Model file for the job. Use its own axes, mm. A direction names the side the tool comes from. Coordinates: 2 decimals unless noted, no trailing zeros. Write each loop counter-clockwise with the first axis right and the second up, starting at its lowest first coordinate (ties: lowest second). Pieces come first, ordered by that corner, then holes. Notation, with made-up numbers: M 51.5,56.5 L 104.5,56.5 A21 ccw 104.5,76.5 Z; hole C 51.5,-25 d11. An arc over 180 degrees is marked long. One line per question, with ' | ' between items. Start each with the question number.
(1) Flat gauge pins, fed straight in: pin 1 Ø6 at (y, z) = (-5, 5) entering from +X; pin 2 Ø1.5 at (y, z) = (-6.5, 5) entering from +X. Where does each tip first touch, or does it go through?
(2) Cut at A-A (x = 8). Write the cut outline in (y, z).
(3) Cut at D-D (z = 1.5). Write the cut outline in (x, y), plus the area to 3 significant figures.
(4) Two-plate mould, pull along Z, no slides. Class faces 3 (the face through (-6, -10, 5)), 4 (the face through (0, -5, 10)), 5 (the face through (-6.04, -3.66, 7.11)): +Z half, -Z half, draft (parallel to the pull), parting line (faces both ways), or undercut.
(5) Wall check: probe 1 along Y at (x, z) = (5, 5); probe 2 along Z at (x, y) = (0, -6.6); probe 3 along X at (y, z) = (-8.5, 6.25). Give the ranges that are in metal, low to high.
(6) Tool access for faces 1 (the face through (1.34, -2.85, 7.11)), 2 (the face through (-10, -3, 3)): list every direction of +Z, -Z, +X, -X, +Y, -Y with a clear straight run to the whole face (end or side of a thin tool).
(7) Cut at B-B (z = 5). Write the cut outline in (x, y), plus the area to 3 significant figures.
(8) Cut at C-C (y = -3.25). Write the cut outline in (x, z), plus the area to 3 significant figures.
from build123d import *

# Parameters (mm, degrees)
F0_W          = 20
F0_H          = 10
F1_DEPTH      = 10
F2_R          = 2.5
F3_DEPTH      = 8
F4_R          = 2.5
F5_DEPTH      = 10.001
F5_DEPTH_BACK = 10.001
F6_T1_DEPTH   = 35


# Not quite as in the source:
# - a fillet or chamfer that OpenCascade refuses, or shapes differently, is made with other operations: its cross-section is extruded or revolved along the edge and cut away or added


with BuildPart() as f1:
    # F0 (on Front) → F1 (new body)
    with BuildSketch(Plane.XZ):
        with Locations((0, 5)):
            Rectangle(F0_W, F0_H)
    extrude(amount=F1_DEPTH)

    # F2 (on face) → F3 (cut)
    with BuildSketch(Plane.XZ.offset(10)):
        with Locations((0, 5)):
            Circle(F2_R)
    extrude(amount=-F3_DEPTH, mode=Mode.SUBTRACT)

    # F4 (on Right) → F5 (cut, two sides)
    with BuildSketch(Plane.YZ) as f5_sk:
        with Locations((-5, 5)):
            Circle(F4_R)
    extrude(amount=-F5_DEPTH, mode=Mode.SUBTRACT)
    extrude(f5_sk.sketch, amount=F5_DEPTH_BACK, mode=Mode.SUBTRACT)

    # F6: fillet of radius 3 on 4 edges, made by hand

    # F6_s2 → F6_t1 (cut)
    with BuildSketch(Plane.YZ.offset(-17.5)):
        with BuildLine():
            ThreePointArc((-3, 10), (-0.8786796564, 9.1213203436), (0, 7))
            Line((0, 7), (0, 10))
            Line((0, 10), (-3, 10))
        make_face()
        with BuildLine():
            ThreePointArc((-7, 10), (-9.1213203436, 9.1213203436), (-10, 7))
            Line((-10, 7), (-10, 10))
            Line((-10, 10), (-7, 10))
        make_face()
        with BuildLine():
            ThreePointArc((-10, 3), (-9.1213203436, 0.8786796564), (-7, 0))
            Line((-7, 0), (-10, 0))
            Line((-10, 0), (-10, 3))
        make_face()
        with BuildLine():
            ThreePointArc((0, 3), (-0.8786796564, 0.8786796564), (-3, 0))
            Line((-3, 0), (0, 0))
            Line((0, 0), (0, 3))
        make_face()
    extrude(amount=F6_T1_DEPTH, mode=Mode.SUBTRACT)


solid = f1.part
Filled in:
1) pin 1: x = 10 | pin 2: through
2) outline: M -10,3 A3 ccw -7,0 L -3,0 A3 ccw 0,3 L 0,7 A3 ccw -3,10 L -7,10 A3 ccw -10,7 Z; hole C -5,5 d5
3) outline: M -10,-9.6 L 10,-9.6 L 10,-0.4 L -10,-0.4 Z | area: 184 mm²
4) face 3: draft | face 4: +Z half | face 5: undercut
5) probe 1: -10 to -7.5, -2.5 to 0 | probe 2: 0 to 2.5, 7.5 to 10 | probe 3: -10 to -2.17, 2.17 to 10
6) face 1: -Y | face 2: +Z, -Z, -X, +Y, -Y
7) outline: M -10,-10 L -2.5,-10 L -2.5,-7.5 L -10,-7.5 Z; M -10,-2.5 L -2.5,-2.5 L -2.5,-2 L 2.5,-2 L 2.5,-2.5 L 10,-2.5 L 10,0 L -10,0 Z; M 2.5,-10 L 10,-10 L 10,-7.5 L 2.5,-7.5 Z | area: 85.0 mm²
8) outline: M -10,0 L 10,0 L 10,3.21 L 1.75,3.21 A2.5 cw -1.75,3.21 L -10,3.21 Z; M -10,6.79 L -1.75,6.79 A2.5 cw 1.75,6.79 L 10,6.79 L 10,10 L -10,10 Z | area: 125 mm²
